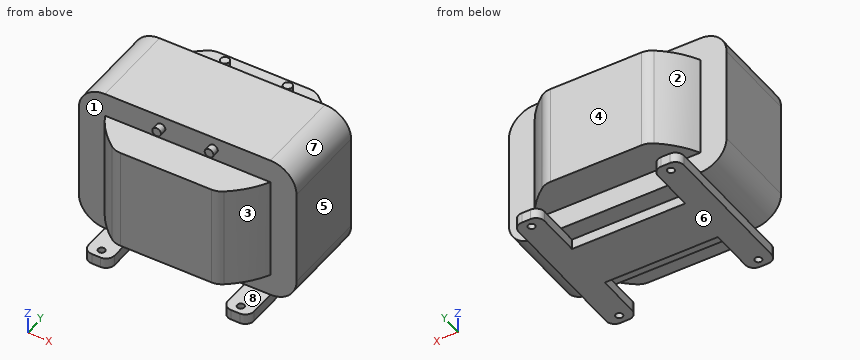
Solid Edge part; units mm, degrees
sketch "Sketch1" plane through (0, 0, 0) normal (0, 0, 1) x (1, 0, 0)
  line L0 (-45.4008, 17.7946) -> (79.5992, 17.7946)
  line L1 (79.5992, 17.7946) -> (79.5992, 67.7946)
  line L2 (79.5992, 67.7946) -> (-45.4008, 67.7946)
  line L3 (-45.4008, 67.7946) -> (-45.4008, 17.7946)
extrude "Protrusion1" add sketch "Sketch1" along normal blind 85
fillet "Round_1" radius 15 4 edges at (79.5992, 42.7946, 85) (-45.4008, 42.7946, 85) (-45.4008, 42.7946, 0) (79.5992, 42.7946, 0)
sketch "Sketch2" plane through (0, 0, 12.5) normal (0, 0, 1) x (1, 0, 0)
  line L0 (64.5992, 67.7946) -> (-30.4008, 67.7946)
  arc A0 (-30.4008, 67.7946) -> (64.5992, 67.7946) centre (17.0992, 42.7946) cw
  line L1 (-30.4008, 17.7946) -> (64.5992, 17.7946)
  arc A1 (64.5992, 17.7946) -> (-30.4008, 17.7946) centre (17.0992, 42.7946) cw
  dimension "D1" = 64.5992
extrude "ExtrudedProtrusion_2" add sketch "Sketch2" along normal blind 58.8
sketch "Sketch3" plane through (17.0992, 82.1333, 71.3) normal (0, 0, 1) x (-1, 0, 0)
  line L0 (-62.5, -5.6614) -> (69.2147, -5.6614)
extrude "Cutout1" cut sketch "Sketch3" against normal through all material side at (13.7418, 87.8447, 71.3)
sketch "Sketch4" plane through (17.0992, 3.456, 71.3) normal (0, 0, 1) x (-1, 0, 0)
  line L0 (-65.9867, 5.6614) -> (63.9181, 5.6614)
extrude "Cutout2" cut sketch "Sketch4" against normal through all material side at (18.1335, -2.2554, 71.3)
fillet "Round_2" radius 10 4 edges at (46.361, 87.7946, 41.9) (-12.1625, 87.7946, 41.9) (-12.1625, -2.2054, 41.9) (46.361, -2.2054, 41.9)
sketch "Sketch5" plane through (17.0992, 42.7946, 0) normal (0, 0, -1) x (-1, 0, 0)
  line L0 (-32.5, 45) -> (-47.5, 45)
  line L1 (-47.5, -45) -> (-47.5, 45)
  line L2 (-32.5, -45) -> (-47.5, -45)
  line L3 (-32.5, -45) -> (-32.5, -15)
  line L4 (32.5, -15) -> (-32.5, -15)
  line L5 (32.5, -15) -> (32.5, -45)
  line L6 (32.5, -45) -> (47.5, -45)
  line L7 (47.5, 45) -> (47.5, -45)
  line L8 (47.5, 45) -> (32.5, 45)
  line L9 (32.5, 45) -> (32.5, 15)
  line L10 (32.5, 15) -> (-32.5, 15)
  line L11 (-32.5, 15) -> (-32.5, 45)
extrude "ExtrudedProtrusion_3" add sketch "Sketch5" along normal blind 6
fillet "Round_3" radius 5 8 edges at (64.5992, -2.2054, -3) (49.5992, -2.2054, -3) (-15.4008, -2.2054, -3) (-30.4008, -2.2054, -3) (64.5992, 87.7946, -3) (49.5992, 87.7946, -3) (-30.4008, 87.7946, -3) (-15.4008, 87.7946, -3)
sketch "Sketch6" plane through (57.0992, 77.7946, 0) normal (0, 0, 1) x (0, -1, 0)
  circle A0 centre (-5, 0) radius 2
  circle A1 centre (75, -0.0992) radius 2
  circle A2 centre (-5, -80) radius 2
  circle A3 centre (75, -80) radius 2
extrude "Cutout3" cut sketch "Sketch6" against normal through all
sketch "Sketch7" plane through (17.0992, 17.7946, 42.5) normal (0, -1, 0) x (1, 0, 0)
  circle A0 centre (-15.3327, 35.4738) radius 2.5
  circle A1 centre (14.7883, 35.4738) radius 2.5
extrude "ExtrudedProtrusion_4" add sketch "Sketch7" along normal blind 4
sketch "Sketch8" plane through (17.0992, 77.7946, 71.3) normal (0, 0, 1) x (1, 0, 0)
  circle A0 centre (-18.4101, 3.3786) radius 2.5
  circle A1 centre (17.7206, 3.3786) radius 2.5
extrude "ExtrudedProtrusion_5" add sketch "Sketch8" along normal blind 3.175
Source: CAD feature listing. Evaluate the final solid. Frame: model axes, mm. Face numbers are marked on the shaded views. A direction names the side the tool comes from. Round coordinates to 2 decimals unless told otherwise and drop trailing zeros. Write each loop counter-clockwise with the first axis right and the second up, starting at its lowest first coordinate (ties: lowest second). Pieces come first, ordered by that corner, then holes. Notation, with made-up numbers: (-34.75, 7.25) - (-28.75, 7.25) arc R33 ccw to (-28.75, 38.25) - close; hole circle Ø5 at (31.25, -26.5). An arc over 180 degrees is marked (long way). Use CSV: the item, a comma, the result in double quotes. Start each with the question number.
(1) Cut plane C-C, the plane y = 49. Return loops of the section in (x, z).
(2) Cut plane A-A, the plane x = 19. Return loops of the section in (y, z).
(3) Cut plane B-B, the plane z = 63. Return loops of the section in (x, y).
(4) First-contact query: pin 1 Ø8 at (x, z) = (38, 8) entering from -Y; pin 2 Ø6 at (x, y) = (32, 77.5) entering from +Z (3 decimals); pin 3 Ø4.5 at (x, y) = (57, 2.79) entering from +Z; pin 4 Ø3.5 at (x, y) = (-22.9, 2.79) entering from -Z. Flat tips, straight axial feed; report the tip coordinate or a pass-through.
(5) Cut plane D-D, the plane y = 63. Return loops of the section in (x, z).
(6) Material intervals for probe 1 along Z at (x, y) = (65, 47); probe 2 along Z at (x, y) = (22.5, 6.5); probe 3 along Y at (x, z) = (-36.5, 22), sorted ascending. Write a range as [from, to].
(7) Mould query, pull axis Z, two halves, no side actions, for the marked faces 5, 6, 7 and 8. Classes: pulls with the +Z half, pulls with the -Z half, needs draft (parallel to the pull), parting line crosses it, or undercut.
(8) Set-up query: the marked faces 1, 2, 3 and 4. Return all of +Z, -Z, +X, -X, +Y, -Y with unobstructed straight access to the full face (end or side cutting, diameter ignored); none if empty.
Geometry says:
1,outline,"(-45.4, 15) arc R15 ccw to (-30.4, 0) - (-30.4, -6) - (64.6, -6) - (64.6, 0) arc R15 ccw to (79.6, 15) - (79.6, 70) arc R15 ccw to (64.6, 85) - (-30.4, 85) arc R15 ccw to (-45.4, 70) - close"
2,outline,"(-2.21, 12.5) - (17.79, 12.5) - (17.79, 0) - (27.79, 0) - (27.79, -6) - (57.79, -6) - (57.79, 0) - (67.79, 0) - (67.79, 12.5) - (87.79, 12.5) - (87.79, 71.3) - (67.79, 71.3) - (67.79, 85) - (17.79, 85) - (17.79, 71.3) - (-2.21, 71.3) - close"
3,outline,"(-45.4, 17.79) - (-30.4, 17.79) arc R53.68 ccw to (-15.01, -0.22) arc R10 ccw to (-9.03, -2.21) - (43.23, -2.21) arc R10 ccw to (49.21, -0.22) arc R53.68 ccw to (64.6, 17.79) - (79.6, 17.79) - (79.6, 67.79) - (64.6, 67.79) arc R53.68 ccw to (49.21, 85.81) arc R10 ccw to (43.23, 87.79) - (-9.03, 87.79) arc R10 ccw to (-15.01, 85.81) arc R53.68 ccw to (-30.4, 67.79) - (-45.4, 67.79) - close"
4,pin 1,"y = 17.79"
4,pin 2,"z = 74.475"
4,pin 3,"z = 0"
4,pin 4,"through"
5,outline,"(-45.4, 15) arc R15 ccw to (-30.4, 0) - (-30.4, -6) - (-15.4, -6) - (-15.4, 0) - (49.6, 0) - (49.6, -6) - (64.6, -6) - (64.6, 0) arc R15 ccw to (79.6, 15) - (79.6, 70) arc R15 ccw to (64.6, 85) - (-30.4, 85) arc R15 ccw to (-45.4, 70) - close"
6,probe 1,"[0.01, 84.99]"
6,probe 2,"[12.5, 71.3]"
6,probe 3,"[17.79, 67.79]"
7,face 5,"needs draft"
7,face 6,"pulls with the -Z half"
7,face 7,"pulls with the +Z half"
7,face 8,"undercut"
8,face 1,"-Y"
8,face 2,"+Z, -X, +Y"
8,face 3,"+Z, +X, -Y"
8,face 4,"+Z, -Z, +X, -X, +Y"
